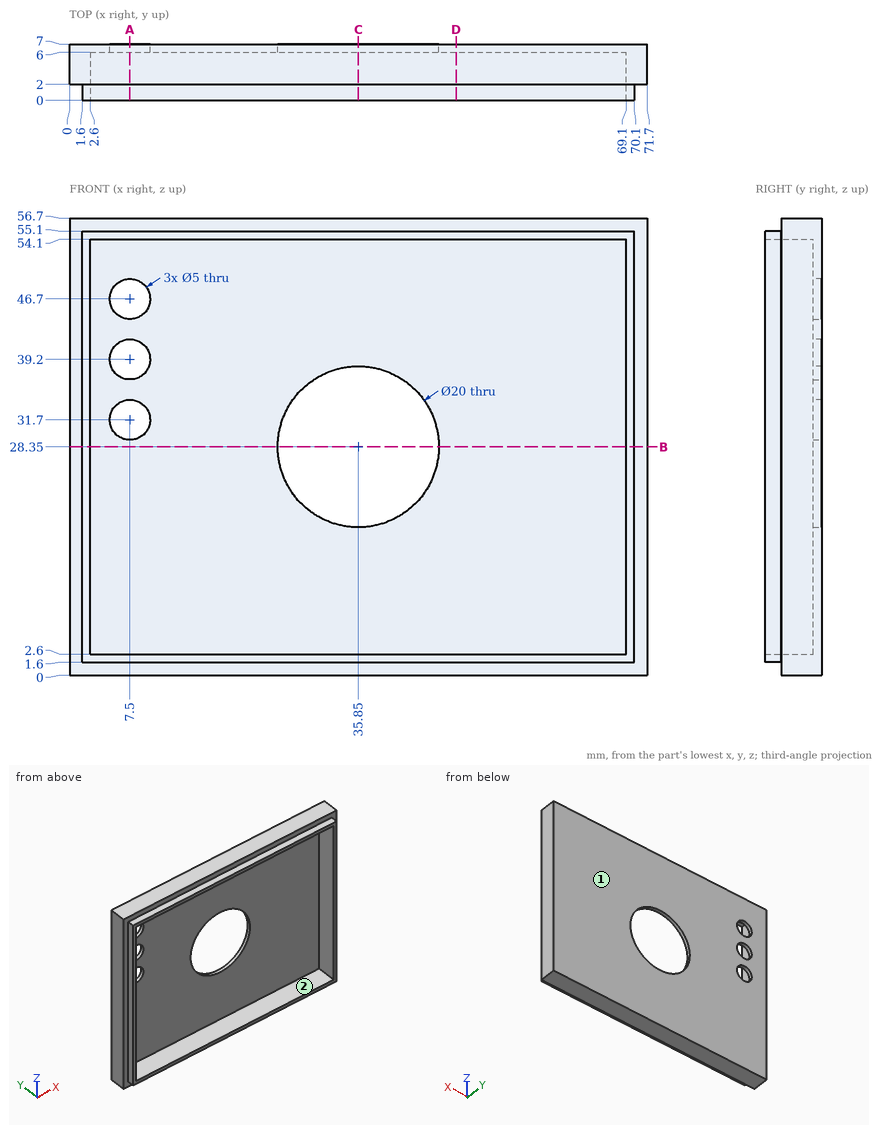
Can you work these out from the drawing? Everything is in mm from the part's minimum corner. Coordinates: 2 decimals unless noted, no trailing zeros. Loops run counter-clockwise (first coordinate to the right, second up) from the corner with the lowest first, then second, coordinate; pieces in that order, holes last.
1. If we mould it in two halves opening along X, with no side actions, what happens to the marked faces 1 and 2? For each: pulls with the +X half, pulls with the -X half, needs draft (parallel to the pull), parting line crosses it, or undercut.
2. Imagine slicing it at D-D, the plane x = 48. Please give me the cut outline in (y, z).
3. Imagine slicing it at B-B, the plane z = 28.35. Please give me the cut outline in (x, y), and give its area (3 significant figures).
4. Imagine slicing it at C-C, the plane x = 35.85. Please give me the cut outline in (y, z), and give its area (3 significant figures).
5. Imagine slicing it at A-A, the plane x = 7.5. Please give me the cut outline in (y, z).
6. For P1, Ø4, axis at x = 23, z = 8.5, coming from the -Y side; P2, Ø4, axis at x = 13, y = 3.5, coming from the -Z side; P3, Ø1.6, axis at y = 1, z = 16.5, coming from the +X side; P4, Ø1.6, axis at x = 51, y = 1, coming from the +Z side, each with a flat end and sliding along its axis, tell me the tip position at first contact or that it passes through.
7. I need wall thicknesses on L1, parallel to X at y = 6.7, z = 28.35; L2, parallel to Z at x = 44, y = 1.25; L3, parallel to X at y = 0.5, z = 6. Which ranges of each line are inside material? Lowest first, please.
Taken from the geometry:
1. face 1: needs draft
1. face 2: undercut
2. outline: (0, 1.6) - (2, 1.6) - (2, 0) - (7, 0) - (7, 56.7) - (2, 56.7) - (2, 55.1) - (0, 55.1) - (0, 54.1) - (6, 54.1) - (6, 2.6) - (0, 2.6) - close
3. outline: (0, 2) - (1.6, 2) - (1.6, 0) - (2.6, 0) - (2.6, 6) - (25.85, 6) - (25.85, 7) - (0, 7) - close; (45.85, 6) - (69.1, 6) - (69.1, 0) - (70.1, 0) - (70.1, 2) - (71.7, 2) - (71.7, 7) - (45.85, 7) - close
3. area: 76.5 mm2
4. outline: (0, 1.6) - (2, 1.6) - (2, 0) - (7, 0) - (7, 18.35) - (6, 18.35) - (6, 2.6) - (0, 2.6) - close; (0, 54.1) - (6, 54.1) - (6, 38.35) - (7, 38.35) - (7, 56.7) - (2, 56.7) - (2, 55.1) - (0, 55.1) - close
4. area: 61.5 mm2
5. outline: (0, 1.6) - (2, 1.6) - (2, 0) - (7, 0) - (7, 29.2) - (6, 29.2) - (6, 2.6) - (0, 2.6) - close; (0, 54.1) - (6, 54.1) - (6, 49.2) - (7, 49.2) - (7, 56.7) - (2, 56.7) - (2, 55.1) - (0, 55.1) - close; (6, 34.2) - (7, 34.2) - (7, 36.7) - (6, 36.7) - close; (6, 41.7) - (7, 41.7) - (7, 44.2) - (6, 44.2) - close
6. P1: stops at y = 6
6. P2: stops at z = 0
6. P3: stops at x = 70.1
6. P4: stops at z = 55.1
7. L1: x = 0 to 25.85, 45.85 to 71.7
7. L2: z = 1.6 to 2.6, 54.1 to 55.1
7. L3: x = 1.6 to 2.6, 69.1 to 70.1
